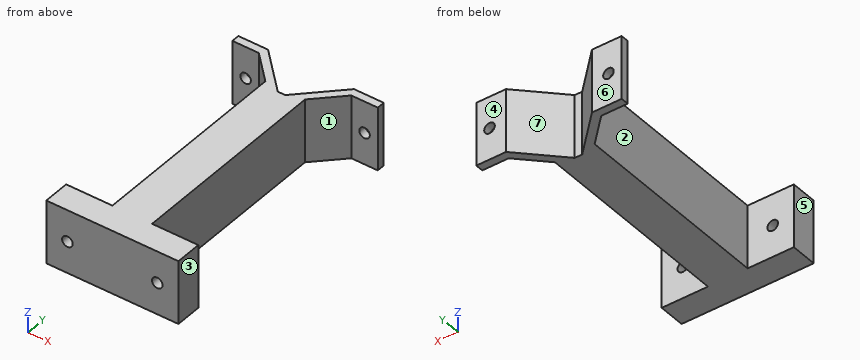
Autodesk Inventor part; units mm, degrees
ref_plane "YZ Plane" through (0, 0, 0) normal (1, 0, 0) x (0, 1, 0)
ref_plane "XZ Plane" through (0, 0, 0) normal (0, 1, 0) x (-1, 0, 0)
ref_plane "XY Plane" through (0, 0, 0) normal (0, 0, 1) x (1, 0, 0)
sketch "Sketch1" plane through (0, 0, 0) normal (0, 0, 1) x (1, 0, 0)
  line L0 (0, -124.1012) -> (0, 44.6073)
  line L1 (0, 44.6073) -> (0, -124.1012)
  line L2 (-38.5085, 0) -> (38.5085, 0)
  line L3 (0, -16.2635) -> (16.2635, 0)
  line L4 (16.2635, 0) -> (0, 16.2635)
  line L5 (0, 16.2635) -> (-16.2635, 0)
  line L6 (-16.2635, 0) -> (0, -16.2635)
  line L7 (0, -16.2635) -> (0, 16.2635) construction
  line L8 (16.2635, 0) -> (-16.2635, 0) construction
  line L9 (0, -16.2635) -> (23, -16.2635) construction
  line L10 (0, -20.5061) -> (-17.5061, -3)
  line L11 (-17.5061, -3) -> (-27.5061, -3)
  line L12 (-27.5061, -3) -> (-27.5061, 3)
  line L13 (-27.5061, 3) -> (-17.5061, 3)
  line L14 (-17.5061, 3) -> (0, 20.5061)
  line L15 (0, 20.5061) -> (17.5061, 3)
  line L16 (17.5061, -3) -> (0, -20.5061)
  line L17 (-38.5085, 0) -> (38.5085, 0)
  line L18 (-27.5061, 0) -> (-16.2635, 0)
  line L19 (16.2635, 0) -> (23.5061, 0)
  line L20 (17.5061, -3) -> (27.5061, -3)
  line L21 (27.5061, -3) -> (27.5061, 3)
  line L22 (27.5061, 3) -> (17.5061, 3)
  line L23 (16.2635, 0) -> (27.5061, 0)
  line L24 (-7.5, -13.0061) -> (-7.5, -90)
  line L25 (-7.5, -90) -> (-25, -90)
  line L26 (-25, -90) -> (-25, -100)
  line L27 (-25, -100) -> (25, -100)
  line L28 (25, -100) -> (25, -90)
  line L29 (25, -90) -> (7.5, -90)
  line L30 (7.5, -90) -> (7.5, -13.0061)
  point P0 (0, 0)
  point P1 (-16.2635, 0)
  point P2 (16.2635, 0)
  point P3 (27.5061, 0)
  point P4 (16.2635, 0)
  point P5 (-16.2635, 0)
  dimension "d34" = 23
  dimension "d35" = 45
  dimension "d36" = 23
  dimension "d37" = 3
  dimension "d38" = 3
  dimension "d39" = 45
  dimension "d41" = 6
  dimension "d49" = 10
  dimension "d50" = 6
  dimension "d51" = 3
  dimension "d52" = 10
  dimension "d69" = 15
  dimension "d70" = 50
  dimension "d71" = 10
  dimension "d72" = 100
extrude "Extrusion3" add sketch "Sketch1" along normal blind 24 contours L10 L11 L12 L2 L6 L0 | L16 L30 L29 L28 L27 L0 | L0 L27 L26 L25 L24 L10 | L0 L3 L2 L21 L20 L16
sketch "Sketch4" plane through (-27.5061, 0, 0) normal (0, 1, 0) x (1, 0, 0)
  line L0 (11.2426, 0) -> (0, 0)
  line L1 (55.0122, 0) -> (43.7696, 0)
  line L2 (0, 0) -> (0, -24)
  line L3 (55.0122, 0) -> (55.0122, -24)
  point P0 (27.5061, 0)
  point P1 (5, -12)
  point P2 (50.0122, -12)
  dimension "d75" = 12
  dimension "d76" = 12
  dimension "d77" = 5
  dimension "d78" = 5
hole "Hole2" at (-22.5061, 0, 12) at (22.5061, 0, 12) direction (0, -1, 0) diameter 4 depth 3
chamfer "Chamfer2" distance 2 angle 45 1 edges at (0, -16.2635, 12)
sketch "Sketch5" plane through (-25, -100, 0) normal (0, -1, 0) x (1, 0, 0)
  line L0 (-2.5061, 0) -> (-2.5061, 24)
  line L1 (52.5061, 0) -> (52.5061, 24)
  line L2 (0, 24) -> (50, 24)
  line L3 (0, 0) -> (0, 24)
  line L4 (50, 0) -> (50, 24)
  point P0 (25, 0)
  point P1 (8, 12)
  point P2 (42, 12)
  dimension "d91" = 12
  dimension "d92" = 12
  dimension "d93" = 8
  dimension "d94" = 8
hole "Hole3" at (-17, -100, 12) at (17, -100, 12) direction (0, 1, 0) diameter 4 depth 10
properties part number "Fan_bottom_3DPrint"
CAD build for the part. Positions are in the model's coordinates, mm. Face numbers are marked on the shaded views. A direction names the side the tool comes from. Round coordinates to 2 decimals unless told otherwise and drop trailing zeros. Loops run counter-clockwise (first coordinate to the right, second up) from the corner with the lowest first, then second, coordinate; pieces in that order, holes last.
(1) Cut at B-B (y = -7). Give the cut face in (x, z), plus the area to 3 significant figures.
(2) Cut at A-A (z = 12). State how many separate pieces and enclosed holes the cut face has, plus the area to 3 significant figures.
(3) Drop flat-ended pins along their axis: pin 1 (5 mm diameter, centred on y = -92.5, z = 8, fed in from +X); pin 2 (8 mm diameter, centred on y = -93, z = 15.5, fed in from -X); pin 3 (2 mm diameter, centred on x = 14, z = 2.5, fed in from +Y); pin 4 (4 mm diameter, centred on x = 6, y = -88.5, fed in from -Z). Give the stop position or say it passes through.
(4) Cut at C-C (x = 9). Give the cut face in (y, z).
(5) Wall check: line 1 along X through (y, z) = (-93.75, 12); line 2 along Z through (x, y) = (-17, -97.5); line 3 along Y through (x, z) = (-21, 3). Give the ranges that are in metal, low to high.
(6) Cut at D-D (z = 4). Give the cut face in (x, y), plus the area to 3 significant figures.
(7) Which spindle directions (+Z, -Z, +X, -X, +Y, -Y) get a long thin tool onto all of the face, cutting with end or side? Do the marked faces 1, 2, 3 and 4. Say none if no direction does.
(8) Two-plate mould, pull along X, no slides. Class the marked faces 5, 6 and 7: +X half, -X half, draft (parallel to the pull), parting line (faces both ways), or undercut.
Findings below:
1. outline: (-13.51, 0) - (-9.26, 0) - (-9.26, 24) - (-13.51, 24) - close; (9.26, 0) - (13.51, 0) - (13.51, 24) - (9.26, 24) - close
1. area: 204 mm2
2. separate pieces: 5
2. enclosed holes: 0
2. area: 1,700 mm2
3. pin 1: stops at x = 25
3. pin 2: stops at x = -25
3. pin 3: stops at y = -1.26
3. pin 4: stops at z = 0
4. outline: (-100, 0) - (-90, 0) - (-90, 24) - (-100, 24) - close; (-11.51, 0) - (-7.26, 0) - (-7.26, 24) - (-11.51, 24) - close
5. line 1: x = -25 to -19, -15 to 15, 19 to 25
5. line 2: z = 0 to 10, 14 to 24
5. line 3: y = -100 to -90, -3 to 0
6. outline: (-27.51, -3) - (-17.51, -3) - (-7.5, -13.01) - (-7.5, -90) - (-25, -90) - (-25, -100) - (25, -100) - (25, -90) - (7.5, -90) - (7.5, -13.01) - (17.51, -3) - (27.51, -3) - (27.51, 0) - (16.26, 0) - (1.41, -14.85) - (-1.41, -14.85) - (-16.26, 0) - (-27.51, 0) - close
6. area: 1,810 mm2
7. face 1: +Z, -Z, +X
7. face 2: +Z, -Z, -X
7. face 3: +Z, -Z, +X, -Y
7. face 4: +Z, -Z, +X, -X, +Y
8. face 5: -X half
8. face 6: draft
8. face 7: undercut
